```python
from build123d import *

# Parameters (mm, degrees)
SKETCH1_W           = 24
SKETCH1_H           = 10
BOSS_EXTRUDE1_DEPTH = 2
SKETCH2_R           = 1.6
CUT_EXTRUDE1_DEPTH  = 2
SKETCH3_W           = 3
SKETCH3_H           = 8
CUT_EXTRUDE2_DEPTH  = 2


with BuildPart() as part:
    # Sketch1 → Boss-Extrude1 (new body)
    with BuildSketch(Plane.XY):
        with Locations((12, 5)):
            Rectangle(SKETCH1_W, SKETCH1_H)
    extrude(amount=BOSS_EXTRUDE1_DEPTH)

    # Sketch2 → Cut-Extrude1 (cut)
    with BuildSketch(Plane.XY.offset(2)):
        with Locations((4, 5)):
            Circle(SKETCH2_R)
        with Locations((20, 5)):
            Circle(SKETCH2_R)
    extrude(amount=-CUT_EXTRUDE1_DEPTH, mode=Mode.SUBTRACT)

    # Sketch3 → Cut-Extrude2 (cut)
    with BuildSketch(Plane.XY.offset(2)):
        with Locations((12, 5)):
            Rectangle(SKETCH3_W, SKETCH3_H)
    extrude(amount=-CUT_EXTRUDE2_DEPTH, mode=Mode.SUBTRACT)


solid = part.part
```
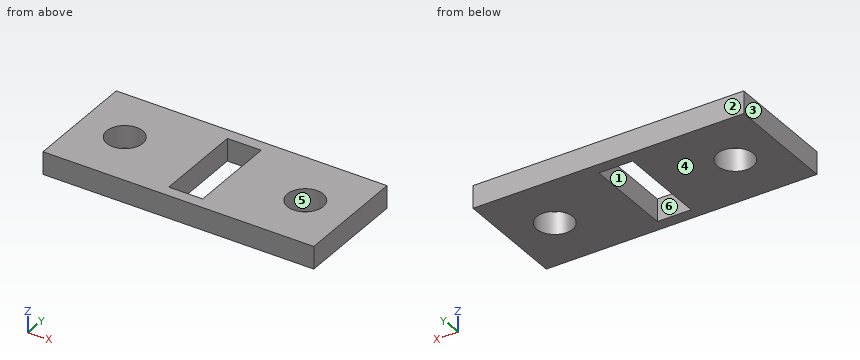
Design review of the part built by this model. Coordinates are the model's own, in mm. Face numbers are marked on the shaded views. A direction names the side the tool comes from. Give positions to 0.01 mm unless a question says otherwise; leave off trailing zeros. Loops run counter-clockwise (first coordinate to the right, second up) from the corner with the lowest first, then second, coordinate; pieces in that order, holes last. Notation, with made-up numbers: (58.5, 56.25) -> (74.5, 56.25) arc R20 cw to (74.5, 73.25) -> close; hole circle Ø9 at (45, 86.5). An arc over 180 degrees is marked (long way). One line per item, written item: value.
Q1. We need section A-A on y = 5. Give the boundary of the cut face in (x, z).
Numbers:
outline: (0, 0) -> (2.4, 0) -> (2.4, 2) -> (0, 2) -> close; (5.6, 0) -> (10.5, 0) -> (10.5, 2) -> (5.6, 2) -> close; (13.5, 0) -> (18.4, 0) -> (18.4, 2) -> (13.5, 2) -> close; (21.6, 0) -> (24, 0) -> (24, 2) -> (21.6, 2) -> close
Q2. We need section B-B on x = 20. Give the boundary of the cut face in (y, z).
Numbers:
outline: (0, 0) -> (3.4, 0) -> (3.4, 2) -> (0, 2) -> close; (6.6, 0) -> (10, 0) -> (10, 2) -> (6.6, 2) -> close
Q3. We need section D-D on z = 0.95. Give the boundary of the cut face in (x, y), and give its area (3 significant figures).
Numbers:
outline: (0, 0) -> (24, 0) -> (24, 10) -> (0, 10) -> close; hole circle Ø3.2 at (4, 5); hole (10.5, 1) -> (13.5, 1) -> (13.5, 9) -> (10.5, 9) -> close; hole circle Ø3.2 at (20, 5)
area: 200 mm^2
Q4. We need section C-C on y = 2.75. Give the boundary of the cut face in (x, z), and give its area (3 significant figures).
Numbers:
outline: (0, 0) -> (10.5, 0) -> (10.5, 2) -> (0, 2) -> close; (13.5, 0) -> (24, 0) -> (24, 2) -> (13.5, 2) -> close
area: 42.0 mm^2
Q5. Machinability: for the marked faces 1 and 2, which of the approach directions +Z, -Z, +X, -X, +Y, -Y give a long, thin tool a straight path to every point of the face, cutting with its end or side? Answer none if there is none.
Numbers:
face 1: +Z, -Z
face 2: +Z, -Z, +X, -X, +Y
Q6. For L1, parallel to Y at x = 20, z = 0.5; L2, parallel to X at y = 7.5, z = 0.7; L3, parallel to Y at x = 12.75, z = 1.9, list the stretches that pass through material, from the lowest coordinate up.
Numbers:
L1: y = 0 to 3.4, 6.6 to 10
L2: x = 0 to 10.5, 13.5 to 24
L3: y = 0 to 1, 9 to 10
Q7. Draft analysis for pull direction X (two halves, no side actions). For the marked faces 3, 4, 5 and 6, state which applies: pulls with the +X half, pulls with the -X half, needs draft (parallel to the pull), parting line crosses it, or undercut.
Numbers:
face 3: pulls with the -X half
face 4: needs draft
face 5: undercut
face 6: undercut
